from build123d import *

# Parameters (mm, degrees)
SKETCH1_R               = 8.001
SKETCH1_R_2             = 6.477
BOSS_EXTRUDE1_DEPTH     = 273.05
CUT_EXTRUDE1_DEPTH      = 9.001
CUT_EXTRUDE1_DEPTH_BACK = 9.001


with BuildPart() as part:
    # Sketch1 → Boss-Extrude1 (new body)
    with BuildSketch(Plane.XY):
        Circle(SKETCH1_R)
        Circle(SKETCH1_R_2, mode=Mode.SUBTRACT)
    extrude(amount=BOSS_EXTRUDE1_DEPTH)

    # Sketch2 → Cut-Extrude1 (cut, two sides)
    with BuildSketch(Plane(origin=(0, 0, 0), x_dir=(0, 0, -1), z_dir=(1, 0, 0))) as cut_extrude1_sk:
        with BuildLine():
            Line((556.557244855, 3.175), (0, 3.175))
            Line((0, 3.175), (-31.75, 3.175))
            ThreePointArc((-31.75, 3.175), (-32.827630735, 2.728630735), (-33.274, 1.651))
            Line((-33.274, 1.651), (-33.274, -1.651))
            ThreePointArc((-33.274, -1.651), (-32.827630735, -2.728630735), (-31.75, -3.175))
            Line((-31.75, -3.175), (0, -3.175))
            Line((0, -3.175), (556.557244855, -3.175))
            Line((556.557244855, -3.175), (1669.671734566, -3.175))
            Line((1669.671734566, -3.175), (1669.671734566, 3.175))
            Line((1669.671734566, 3.175), (556.557244855, 3.175))
        make_face()
    extrude(amount=CUT_EXTRUDE1_DEPTH, mode=Mode.SUBTRACT)
    extrude(cut_extrude1_sk.sketch, amount=-CUT_EXTRUDE1_DEPTH_BACK, mode=Mode.SUBTRACT)


solid = part.part
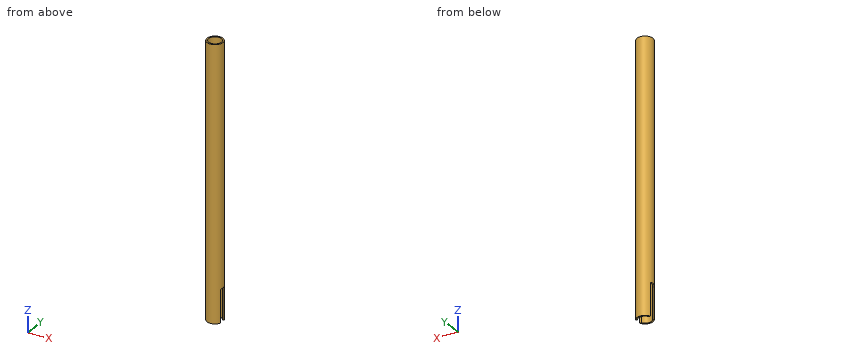
Source: CAD feature listing. Evaluate the final solid. Frame: model axes, mm. Round coordinates to 2 decimals unless told otherwise and drop trailing zeros. Loops run counter-clockwise (first coordinate to the right, second up) from the corner with the lowest first, then second, coordinate; pieces in that order, holes last. Notation, with made-up numbers: (-8.75, -9.5) - (45.25, -9.5) arc R27 ccw to (45.25, 20.5) - close; hole circle Ø4 at (5.5, 54). An arc over 180 degrees is marked (long way). Write item = value, one per line. Start each with the question number.
Item 1: Section query B-B on z = 35.5. Output: boundary loops of the cut face in (x, y).
Item 2: Material intervals for line 1 (X direction, y = -0.25, z = 145); line 2 (Y direction, x = 0, z = 63); line 3 (Y direction, x = 1.5, z = 217.5), sorted ascending.
Item 3: First-contact query: pin 1 Ø1.9 at (x, z) = (6.5, 8) entering from +Y; pin 2 Ø2 at (y, z) = (-5.5, 202) entering from +X; pin 3 Ø1.4 at (x, y) = (-7, 0.5) entering from -Z. Flat tips, straight axial feed; report the tip coordinate or a pass-through.
Item 4: Section query A-A on x = 0. Output: boundary loops of the cut face in (y, z), plus the area to 3 significant figures.
Results list:
q1.outline = circle Ø16 at (0, 0); hole circle Ø12.95 at (0, 0)
q2.line_1 = -8 to -6.47, 6.47 to 8
q2.line_2 = -8 to -6.48, 6.48 to 8
q2.line_3 = -7.86 to -6.3, 6.3 to 7.86
q3.pin_1 = 5.76
q3.pin_2 = 6.62
q3.pin_3 = 33.27
q4.outline = (-8, 0) - (-6.48, 0) - (-6.48, 273.05) - (-8, 273.05) - close; (6.48, 0) - (8, 0) - (8, 273.05) - (6.48, 273.05) - close
q4.area = 832 mm²
